from build123d import *

# Parameters (mm, degrees)
SKETCH2_R           = 9
BOSS_EXTRUDE2_DEPTH = 10
SKETCH3_R           = 8
CUT_EXTRUDE1_DEPTH  = 5
SKETCH4_W           = 4.35
SKETCH4_H           = 6.15
CUT_EXTRUDE2_DEPTH  = 6


with BuildPart() as part:
    # Sketch2 → Boss-Extrude2 (new body)
    with BuildSketch(Plane(origin=(0, 0, 0), x_dir=(1, 0, 0), z_dir=(0, 1, 0))):
        Circle(SKETCH2_R)
    extrude(amount=BOSS_EXTRUDE2_DEPTH)

    # Sketch3 → Cut-Extrude1 (cut)
    with BuildSketch(Plane(origin=(0, 10, 0), x_dir=(1, 0, 0), z_dir=(0, 1, 0))):
        Circle(SKETCH3_R)
    extrude(amount=-CUT_EXTRUDE1_DEPTH, mode=Mode.SUBTRACT)

    # Sketch4 → Cut-Extrude2 (cut, through all)
    with BuildSketch(Plane(origin=(0, 5, 0), x_dir=(1, 0, 0), z_dir=(0, 1, 0))):
        with Locations((-0.006105592, 0)):
            Rectangle(SKETCH4_W, SKETCH4_H)
        with Locations((-4.856105592, 0)):
            Rectangle(SKETCH4_W, SKETCH4_H)
        with Locations((4.843894408, 0)):
            Rectangle(SKETCH4_W, SKETCH4_H)
    extrude(amount=-CUT_EXTRUDE2_DEPTH, mode=Mode.SUBTRACT)


solid = part.part
Could you check a few things on this model? Use its own coordinates, in mm. A direction names the side the tool comes from. Coordinates: 2 decimals unless noted, no trailing zeros. Write each loop counter-clockwise with the first axis right and the second up, starting at its lowest first coordinate (ties: lowest second). Pieces come first, ordered by that corner, then holes. Notation, with made-up numbers: (-2, 76) - (44, 76) arc R33 cw to (44, 106) - close; hole circle Ø3 at (31.25, -10). An arc over 180 degrees is marked (long way). Put each result on its own line as item: value. Start each with the question number.
Q1. I'm going to push flat-ended pins straight in: P1, Ø4, axis at x = -5, z = -1.5, coming from the +Y side; P2, Ø1.3, axis at x = 5, y = 2.5, coming from the -Z side; P3, Ø5, axis at x = 4, y = 2.5, coming from the +Z side. Where does each tip first touch, or does it pass through?
Q2. I want a section at A-A on y = 0.75. Write out the boundary of the cut face in (x, z) (3 decimals).
Q3. Please list where these lines run through material, in increasing order: L1, parallel to Z at x = 0, y = 7.05; L2, parallel to X at y = 1.5, z = -1.5.
Q4. I want a section at D-D on z = 4.75. Write out the boundary of the cut face in (x, y).
Q5. Which directions (+Z, -Z, +X, -X, +Y, -Y) give clear straight access to the entire face, cutting with the end or side of a thin tool? Please do faces 1 (the flat face through (-2.181, 3, 0)), 2 (the cylindrical face through (-1.73, 7.54, 7.81)).
Q6. Thinking about a two-plate mould opening in X: for faces 3 (the flat face through (0, 0, 4)), 4 (the cylindrical face through (-1.172, 4.93, -8.923)), 5 (the flat face through (-2.681, 3, 0)), which applies, pulls with the +X half, pulls with the -X half, needs draft (parallel to the pull), parting line crosses it, or undercut?
Q7. I want a section at B-B on x = 0. Write out the boundary of the cut face in (y, z) (3 decimals), plus the area to 4 significant figures.
Q8. I want a section at C-C on z = 0. Write out the boundary of the cut face in (x, y), plus the area to 4 significant figures.
Checks:
1. P1: y = 5
1. P2: z = -7.88
1. P3: z = 8.87
2. outline: circle Ø18 at (0, 0); hole (-7.031, -3.075) - (-2.681, -3.075) - (-2.681, 3.075) - (-7.031, 3.075) - close; hole (-2.181, -3.075) - (2.169, -3.075) - (2.169, 3.075) - (-2.181, 3.075) - close; hole (2.669, -3.075) - (7.019, -3.075) - (7.019, 3.075) - (2.669, 3.075) - close
3. L1: -9 to -8, 8 to 9
3. L2: -8.87 to -7.03, -2.68 to -2.18, 2.17 to 2.67, 7.02 to 8.87
4. outline: (-7.64, 0) - (7.64, 0) - (7.64, 10) - (6.44, 10) - (6.44, 5) - (-6.44, 5) - (-6.44, 10) - (-7.64, 10) - close
5. face 1: +Y, -Y
5. face 2: +Y
6. face 3: needs draft
6. face 4: parting line crosses it
6. face 5: undercut
7. outline: (0, -9) - (10, -9) - (10, -8) - (5, -8) - (5, -3.075) - (0, -3.075) - close; (0, 3.075) - (5, 3.075) - (5, 8) - (10, 8) - (10, 9) - (0, 9) - close
7. area: 69.25 mm²
8. outline: (-9, 0) - (-7.03, 0) - (-7.03, 5) - (-8, 5) - (-8, 10) - (-9, 10) - close; (-2.68, 0) - (-2.18, 0) - (-2.18, 5) - (-2.68, 5) - close; (2.17, 0) - (2.67, 0) - (2.67, 5) - (2.17, 5) - close; (7.02, 0) - (9, 0) - (9, 10) - (8, 10) - (8, 5) - (7.02, 5) - close
8. area: 34.75 mm²
